The listing builds one solid part. Answer for the finished solid, in the listing's coordinates (mm). A direction names the side the tool comes from. Give positions to 0.01 mm unless a question says otherwise; leave off trailing zeros. Write each loop counter-clockwise with the first axis right and the second up, starting at its lowest first coordinate (ties: lowest second). Pieces come first, ordered by that corner, then holes. Notation, with made-up numbers: M -17.5,-35.5 L 4.5,-35.5 A21 ccw 4.5,-19.5 Z; hole C 1.25,12.5 d2. An arc over 180 degrees is marked long. Return JSON: item names as keys, results as strings.
from build123d import *

# Parameters (mm, degrees)
BOSS_EXTRUDE2_DEPTH  = 38.1
BOSS_EXTRUDE6_DEPTH  = 19.05
SKETCH6_W            = 5.08
SKETCH6_H            = 19.05
BOSS_EXTRUDE5_DEPTH  = 20.32
SKETCH10_W           = 23.1648
SKETCH10_H           = 3.81
SKETCH10_W_2         = 17.5006
CUT_EXTRUDE3_DEPTH   = 19.05
FILLET1_R            = 2.54
BOSS_EXTRUDE7_DEPTH  = 19.05
CLEARANCE_START      = -38.1
SKETCH3_W            = 2.6416
SKETCH3_H            = 20.32
SKETCH3_W_2          = 7.7216
SKETCH3_W_3          = 15.3416
CLEARANCE_TRIM_DEPTH = 38.1


with BuildPart() as part:
    # Sketch1 → Boss-Extrude2 (new body)
    with BuildSketch(Plane.XY):
        with BuildLine():
            Line((-2.016886463, 6.858), (2.016886463, 6.858))
            ThreePointArc((2.016886463, 6.858), (3.83455623, 7.219556996), (5.375502252, 8.249184211))
            Line((5.375502252, 8.249184211), (10.026617928, 12.900299887))
            ThreePointArc((10.026617928, 12.900299887), (10.219328904, 13.188712244), (10.287, 13.528917816))
            Line((10.287, 13.528917816), (10.287, 14.097877816))
            ThreePointArc((10.287, 14.097877816), (10.026617928, 14.726495744), (9.398, 14.986877816))
            Line((9.398, 14.986877816), (4.953, 14.986877816))
            ThreePointArc((4.953, 14.986877816), (4.324382072, 15.247259887), (4.064, 15.875877816))
            Line((4.064, 15.875877816), (4.064, 27.686877816))
            Line((4.064, 27.686877816), (161.036, 27.686877816))
            Line((161.036, 27.686877816), (161.036, 15.875877816))
            ThreePointArc((161.036, 15.875877816), (160.775617928, 15.247259887), (160.147, 14.986877816))
            Line((160.147, 14.986877816), (155.702, 14.986877816))
            ThreePointArc((155.702, 14.986877816), (155.073382072, 14.726495744), (154.813, 14.097877816))
            Line((154.813, 14.097877816), (154.813, 13.528917816))
            ThreePointArc((154.813, 13.528917816), (154.880671096, 13.188712244), (155.073382072, 12.900299887))
            Line((155.073382072, 12.900299887), (159.724497748, 8.249184211))
            ThreePointArc((159.724497748, 8.249184211), (161.26544377, 7.219556996), (163.083113537, 6.858))
            Line((163.083113537, 6.858), (167.116886463, 6.858))
            ThreePointArc((167.116886463, 6.858), (168.93455623, 7.219556996), (170.475502252, 8.249184211))
            Line((170.475502252, 8.249184211), (175.126617928, 12.900299887))
            ThreePointArc((175.126617928, 12.900299887), (175.319328904, 13.188712244), (175.387, 13.528917816))
            Line((175.387, 13.528917816), (175.387, 14.097877816))
            ThreePointArc((175.387, 14.097877816), (175.126617928, 14.726495744), (174.498, 14.986877816))
            Line((174.498, 14.986877816), (170.053, 14.986877816))
            ThreePointArc((170.053, 14.986877816), (169.424382072, 15.247259887), (169.164, 15.875877816))
            Line((169.164, 15.875877816), (169.164, 27.686877816))
            Line((169.164, 27.686877816), (169.164, 34.036877816))
            Line((169.164, 34.036877816), (-4.064, 34.036877816))
            Line((-4.064, 34.036877816), (-4.064, 27.686877816))
            Line((-4.064, 27.686877816), (-4.064, 15.875877816))
            ThreePointArc((-4.064, 15.875877816), (-4.324382072, 15.247259887), (-4.953, 14.986877816))
            Line((-4.953, 14.986877816), (-9.398, 14.986877816))
            ThreePointArc((-9.398, 14.986877816), (-10.026617928, 14.726495744), (-10.287, 14.097877816))
            Line((-10.287, 14.097877816), (-10.287, 13.528917816))
            ThreePointArc((-10.287, 13.528917816), (-10.219328904, 13.188712244), (-10.026617928, 12.900299887))
            Line((-10.026617928, 12.900299887), (-5.375502252, 8.249184211))
            ThreePointArc((-5.375502252, 8.249184211), (-3.83455623, 7.219556996), (-2.016886463, 6.858))
        make_face()
    extrude(amount=BOSS_EXTRUDE2_DEPTH)

    # Sketch7 → Boss-Extrude6 (add)
    with BuildSketch(Plane.XY):
        Polygon((130.81, 106.426877816), (169.164, 106.426877816), (169.164, 110.236877816), (-4.064, 110.236877816), (-4.064, 106.426877816), (34.29, 106.426877816), (34.29, 34.036877816), (38.1, 34.036877816), (38.1, 106.426877816), (127, 106.426877816), (127, 34.036877816), (130.81, 34.036877816), align=None)
    extrude(amount=BOSS_EXTRUDE6_DEPTH)

    # Sketch6 → Boss-Extrude5 (add)
    with BuildSketch(Plane(origin=(0, 110.236877816, 0), x_dir=(1, 0, 0), z_dir=(0, 1, 0))):
        with Locations((21.6408, -9.525)):
            Rectangle(SKETCH6_W, SKETCH6_H)
        with Locations((29.2608, -9.525)):
            Rectangle(SKETCH6_W, SKETCH6_H)
        with Locations((77.5462, -9.525)):
            Rectangle(SKETCH6_W, SKETCH6_H)
        with Locations((90.2462, -9.525)):
            Rectangle(SKETCH6_W, SKETCH6_H)
        with Locations((128.8034, -9.525)):
            Rectangle(SKETCH6_W, SKETCH6_H)
        with Locations((149.1234, -9.525)):
            Rectangle(SKETCH6_W, SKETCH6_H)
    extrude(amount=BOSS_EXTRUDE5_DEPTH)

    # Sketch10 → Cut-Extrude3 (cut)
    with BuildSketch(Plane.XY):
        with Locations((7.5184, 108.331877816)):
            Rectangle(SKETCH10_W, SKETCH10_H)
        with Locations((160.4137, 108.331877816)):
            Rectangle(SKETCH10_W_2, SKETCH10_H)
    extrude(amount=CUT_EXTRUDE3_DEPTH, mode=Mode.SUBTRACT)

    # Fillet1
    fillet1_edges = [part.edges().sort_by_distance(p)[0] for p in [
        (21.6408, 130.556877816, 19.05),
        (21.6408, 130.556877816, 0),
        (29.2608, 130.556877816, 0),
        (29.2608, 130.556877816, 19.05),
        (77.5462, 130.556877816, 0),
        (77.5462, 130.556877816, 19.05),
        (90.2462, 130.556877816, 0),
        (90.2462, 130.556877816, 19.05),
        (128.8034, 130.556877816, 0),
        (128.8034, 130.556877816, 19.05),
        (149.1234, 130.556877816, 0),
        (149.1234, 130.556877816, 19.05),
    ]]
    fillet(fillet1_edges, radius=FILLET1_R)

    # Sketch11 → Boss-Extrude7 (add)
    with BuildSketch(Plane.XY):
        Polygon((38.1, 103.970194938), (79.533021028, 70.231877816), (38.1, 36.493560693), (38.1, 34.036877816), (41.116978972, 34.036877816), (82.55, 67.775194938), (123.983021028, 34.036877816), (127, 34.036877816), (127, 36.493560693), (85.566978972, 70.231877816), (127, 103.970194938), (127, 106.426877816), (123.983021028, 106.426877816), (82.55, 72.688560693), (41.116978972, 106.426877816), (38.1, 106.426877816), align=None)
    extrude(amount=BOSS_EXTRUDE7_DEPTH)

    # Sketch3 → Clearance Trim (cut)
    with BuildSketch(Plane.XY.offset(38.1).offset(CLEARANCE_START)):
        with BuildLine():
            Line((4.064, 27.686877816), (3.937, 21.336877816))
            Line((3.937, 21.336877816), (3.937, 15.875877816))
            ThreePointArc((3.937, 15.875877816), (4.23457951, 15.157457326), (4.953, 14.859877816))
            Line((4.953, 14.859877816), (9.398, 14.859877816))
            ThreePointArc((9.398, 14.859877816), (9.936815367, 14.636693183), (10.16, 14.097877816))
            Line((10.16, 14.097877816), (10.16, 13.528917816))
            ThreePointArc((10.16, 13.528917816), (10.101996204, 13.23731304), (9.936815367, 12.990102448))
            Line((9.936815367, 12.990102448), (5.285699691, 8.338986772))
            ThreePointArc((5.285699691, 8.338986772), (3.785955434, 7.336889697), (2.016886463, 6.985))
            Line((2.016886463, 6.985), (-2.016886463, 6.985))
            ThreePointArc((-2.016886463, 6.985), (-3.785955434, 7.336889697), (-5.285699691, 8.338986772))
            Line((-5.285699691, 8.338986772), (-9.936815367, 12.990102448))
            ThreePointArc((-9.936815367, 12.990102448), (-10.101996204, 13.23731304), (-10.16, 13.528917816))
            Line((-10.16, 13.528917816), (-10.16, 14.097877816))
            ThreePointArc((-10.16, 14.097877816), (-9.936815367, 14.636693183), (-9.398, 14.859877816))
            Line((-9.398, 14.859877816), (-4.953, 14.859877816))
            ThreePointArc((-4.953, 14.859877816), (-4.23457951, 15.157457326), (-3.937, 15.875877816))
            Line((-3.937, 15.875877816), (-3.937, 21.336877816))
            Line((-3.937, 21.336877816), (-4.064, 27.686877816))
            Line((-4.064, 27.686877816), (-4.064, 15.875877816))
            ThreePointArc((-4.064, 15.875877816), (-4.324382072, 15.247259887), (-4.953, 14.986877816))
            Line((-4.953, 14.986877816), (-9.398, 14.986877816))
            ThreePointArc((-9.398, 14.986877816), (-10.026617928, 14.726495744), (-10.287, 14.097877816))
            Line((-10.287, 14.097877816), (-10.287, 13.528917816))
            ThreePointArc((-10.287, 13.528917816), (-10.219328904, 13.188712244), (-10.026617928, 12.900299887))
            Line((-10.026617928, 12.900299887), (-5.375502252, 8.249184211))
            ThreePointArc((-5.375502252, 8.249184211), (-3.83455623, 7.219556996), (-2.016886463, 6.858))
            Line((-2.016886463, 6.858), (2.016886463, 6.858))
            ThreePointArc((2.016886463, 6.858), (3.83455623, 7.219556996), (5.375502252, 8.249184211))
            Line((5.375502252, 8.249184211), (10.026617928, 12.900299887))
            ThreePointArc((10.026617928, 12.900299887), (10.219328904, 13.188712244), (10.287, 13.528917816))
            Line((10.287, 13.528917816), (10.287, 14.097877816))
            ThreePointArc((10.287, 14.097877816), (10.026617928, 14.726495744), (9.398, 14.986877816))
            Line((9.398, 14.986877816), (4.953, 14.986877816))
            ThreePointArc((4.953, 14.986877816), (4.324382072, 15.247259887), (4.064, 15.875877816))
            Line((4.064, 15.875877816), (4.064, 27.686877816))
        make_face()
        with BuildLine():
            Line((161.036, 27.686877816), (161.163, 21.336877816))
            Line((161.163, 21.336877816), (161.163, 15.875877816))
            ThreePointArc((161.163, 15.875877816), (160.86542049, 15.157457326), (160.147, 14.859877816))
            Line((160.147, 14.859877816), (155.702, 14.859877816))
            ThreePointArc((155.702, 14.859877816), (155.163184633, 14.636693183), (154.94, 14.097877816))
            Line((154.94, 14.097877816), (154.94, 13.528917816))
            ThreePointArc((154.94, 13.528917816), (154.998003796, 13.23731304), (155.163184633, 12.990102448))
            Line((155.163184633, 12.990102448), (159.814300309, 8.338986772))
            ThreePointArc((159.814300309, 8.338986772), (161.314044566, 7.336889697), (163.083113537, 6.985))
            Line((163.083113537, 6.985), (167.116886463, 6.985))
            ThreePointArc((167.116886463, 6.985), (168.885955434, 7.336889697), (170.385699691, 8.338986772))
            Line((170.385699691, 8.338986772), (175.036815367, 12.990102448))
            ThreePointArc((175.036815367, 12.990102448), (175.201996204, 13.23731304), (175.26, 13.528917816))
            Line((175.26, 13.528917816), (175.26, 14.097877816))
            ThreePointArc((175.26, 14.097877816), (175.036815367, 14.636693183), (174.498, 14.859877816))
            Line((174.498, 14.859877816), (170.053, 14.859877816))
            ThreePointArc((170.053, 14.859877816), (169.33457951, 15.157457326), (169.037, 15.875877816))
            Line((169.037, 15.875877816), (169.037, 21.336877816))
            Line((169.037, 21.336877816), (169.164, 27.686877816))
            Line((169.164, 27.686877816), (169.164, 15.875877816))
            ThreePointArc((169.164, 15.875877816), (169.424382072, 15.247259887), (170.053, 14.986877816))
            Line((170.053, 14.986877816), (174.498, 14.986877816))
            ThreePointArc((174.498, 14.986877816), (175.126617928, 14.726495744), (175.387, 14.097877816))
            Line((175.387, 14.097877816), (175.387, 13.528917816))
            ThreePointArc((175.387, 13.528917816), (175.319328904, 13.188712244), (175.126617928, 12.900299887))
            Line((175.126617928, 12.900299887), (170.475502252, 8.249184211))
            ThreePointArc((170.475502252, 8.249184211), (168.93455623, 7.219556996), (167.116886463, 6.858))
            Line((167.116886463, 6.858), (163.083113537, 6.858))
            ThreePointArc((163.083113537, 6.858), (161.26544377, 7.219556996), (159.724497748, 8.249184211))
            Line((159.724497748, 8.249184211), (155.073382072, 12.900299887))
            ThreePointArc((155.073382072, 12.900299887), (154.880671096, 13.188712244), (154.813, 13.528917816))
            Line((154.813, 13.528917816), (154.813, 14.097877816))
            ThreePointArc((154.813, 14.097877816), (155.073382072, 14.726495744), (155.702, 14.986877816))
            Line((155.702, 14.986877816), (160.147, 14.986877816))
            ThreePointArc((160.147, 14.986877816), (160.775617928, 15.247259887), (161.036, 15.875877816))
            Line((161.036, 15.875877816), (161.036, 27.686877816))
        make_face()
        with Locations((25.4508, 120.396877816)):
            Rectangle(SKETCH3_W, SKETCH3_H)
        with Locations((83.8962, 120.396877816)):
            Rectangle(SKETCH3_W_2, SKETCH3_H)
        with Locations((138.9634, 120.396877816)):
            Rectangle(SKETCH3_W_3, SKETCH3_H)
    extrude(amount=CLEARANCE_TRIM_DEPTH, mode=Mode.SUBTRACT)


solid = part.part
Item 1: Given pin 1 Ø4.5 at (y, z) = (18, 14) entering from +X; pin 2 Ø1 at (y, z) = (48.5, 8.5) entering from -X; pin 3 Ø2 at (x, z) = (84.5, 22.5) entering from -Y, each flat-ended and moving along its own axis, determine where each tip first touches the part or whether it passes through.
Geometry results:
{"pin 1": "stops at x = 169.04", "pin 2": "stops at x = 34.29", "pin 3": "stops at y = 27.69"}
Item 2: A cutting plane is placed at C-C, the plane y = 58. Write down the section's boundary in (x, z).
Geometry results:
{"outline": "M 34.29,0 L 38.1,0 L 38.1,19.05 L 34.29,19.05 Z; M 64.51,0 L 70.55,0 L 70.55,19.05 L 64.51,19.05 Z; M 94.55,0 L 100.59,0 L 100.59,19.05 L 94.55,19.05 Z; M 127,0 L 130.81,0 L 130.81,19.05 L 127,19.05 Z"}
Item 3: A cutting plane is placed at A-A, the plane x = 29. Write down the section's boundary in (y, z).
Geometry results:
{"outline": "M 27.69,0 L 34.04,0 L 34.04,38.1 L 27.69,38.1 Z; M 106.43,0 L 128.02,0 A2.54 ccw 130.56,2.54 L 130.56,16.51 A2.54 ccw 128.02,19.05 L 106.43,19.05 Z"}
Item 4: A cutting plane is placed at B-B, the plane y = 117. Write down the section's boundary in (x, z), plus the area to 3 significant figures.
Geometry results:
{"outline": "M 19.1,0 L 24.13,0 L 24.13,19.05 L 19.1,19.05 Z; M 26.77,0 L 31.8,0 L 31.8,19.05 L 26.77,19.05 Z; M 75.01,0 L 80.04,0 L 80.04,19.05 L 75.01,19.05 Z; M 87.76,0 L 92.79,0 L 92.79,19.05 L 87.76,19.05 Z; M 126.26,0 L 131.29,0 L 131.29,19.05 L 126.26,19.05 Z; M 146.63,0 L 151.66,0 L 151.66,19.05 L 146.63,19.05 Z", "area": "575 mm2"}
Item 5: Find the intervals of material crossed by line 1 (X direction, y = 120.5, z = 6.5); line 2 (X direction, y = 57.5, z = 14); line 3 (Y direction, x = 74, z = 6.5), in increasing order.
Geometry results:
{"line 1": "x = 19.1 to 24.13, 26.77 to 31.8, 75.01 to 80.04, 87.76 to 92.79, 126.26 to 131.29, 146.63 to 151.66", "line 2": "x = 34.29 to 38.1, 63.9 to 69.93, 95.17 to 101.2, 127 to 130.81", "line 3": "y = 27.69 to 34.04, 60.81 to 65.73, 74.74 to 79.65, 106.43 to 110.24"}
Item 6: Which of the six approach directions +Z, -Z, +X, -X, +Y, -Y give full straight-line access (tool end or side, diameter ignored) to faces 4 (the flat face through (31.801, 120, 10)), 5 (the flat face through (75, 78, 19.05)), 6 (the flat face through (169.164, 31, 19)), 7 (the flat face through (82, 106.427, 9)), 8 (the flat face through (27, 106.427, 9))?
Geometry results:
{"face 4": "+Z, -Z, +Y", "face 5": "+Z, +X, -X, +Y", "face 6": "+Z, -Z, +X, +Y", "face 7": "+Z, -Z", "face 8": "+Z, -Z, -X"}
Item 7: A cutting plane is placed at D-D, the plane z = 7. Count the separate pieces of the cut face and the enclosed holes in it, plus the area to 3 significant figures.
Geometry results:
{"separate pieces": "1", "enclosed holes": "4", "area": "4,060 mm2"}
Item 8: Determine the mould class of faces 1 (the flat face through (130.81, 70, 9)), 2 (the flat face through (81, 30, 38.1)), 3 (the flat face through (-7, 14.86, 19)) for opening direction Y: +Y half, -Y half, draft (parallel to the pull), parting line (faces both ways), or undercut.
Geometry results:
{"face 1": "undercut", "face 2": "draft", "face 3": "+Y half"}
